from build123d import *

# Parameters (mm, degrees)
SKETCH1_R           = 23.87
SKETCH1_R_2         = 1.5875
SKETCH1_R_3         = 1.3208
SKETCH1_R_4         = 4
BOSS_EXTRUDE2_DEPTH = 1.016


with BuildPart() as part:
    # Sketch1 → Boss-Extrude2 (new body)
    with BuildSketch(Plane.XY):
        Circle(SKETCH1_R)
        with Locations((0, 10)):
            Circle(SKETCH1_R_2, mode=Mode.SUBTRACT)
        with Locations((9.878281733, -9.878281733)):
            Circle(SKETCH1_R_3, mode=Mode.SUBTRACT)
        with Locations((9.878281733, 9.878281733)):
            Circle(SKETCH1_R_3, mode=Mode.SUBTRACT)
        with Locations((-9.878281733, -9.878281733)):
            Circle(SKETCH1_R_3, mode=Mode.SUBTRACT)
        with Locations((-9.878281733, 9.878281733)):
            Circle(SKETCH1_R_3, mode=Mode.SUBTRACT)
        Circle(SKETCH1_R_4, mode=Mode.SUBTRACT)
        with Locations((0, -10)):
            Circle(SKETCH1_R_2, mode=Mode.SUBTRACT)
    extrude(amount=BOSS_EXTRUDE2_DEPTH)


solid = part.part
The listing builds one solid part. Answer for the finished solid, in the listing's coordinates (mm). Round coordinates to 2 decimals unless told otherwise and drop trailing zeros. Write each loop counter-clockwise with the first axis right and the second up, starting at its lowest first coordinate (ties: lowest second). Pieces come first, ordered by that corner, then holes. Notation, with made-up numbers: (15.5, 38.25) - (29.5, 38.25) arc R17 cw to (29.5, 59.25) - close; hole circle Ø8 at (65.25, 82). An arc over 180 degrees is marked (long way). Use one line per item in the form item = value. Start each with the question number.
Item 1: A cutting plane is placed at C-C (z = 0.8). Write down the section's boundary in (x, y) (1 decimal).
Item 2: A cutting plane is placed at A-A (x = 0). Write down the section's boundary in (y, z).
Item 3: A cutting plane is placed at D-D (y = -13). Write down the section's boundary in (x, z), plus the area to 3 significant figures.
Item 4: Determine the mould class of faces 1 (the cylindrical face through (0.73, 8.59, 0.5)), 2 (the cylindrical face through (-3.107, 23.667, 0.501)), 3 (the flat face through (5, 0, 1.016)) for opening direction X: +X half, -X half, draft (parallel to the pull), parting line (faces both ways), or undercut.
Item 5: Find the intervals of material crossed by line 1 (Y direction, x = 0, z = 0.2); line 2 (Y direction, x = -1, z = 0.5); line 3 (X direction, y = 9, z = 0.65), in increasing order. Write a range as [from, to].
Item 6: A cutting plane is placed at B-B (y = 0). Write down the section's boundary in (x, z), plus the area to 3 significant figures.
The answers:
q1.outline = circle Ø47.7 at (0, 0); hole circle Ø2.6 at (-9.9, -9.9); hole circle Ø2.6 at (-9.9, 9.9); hole circle Ø8 at (0, 0); hole circle Ø3.2 at (0, -10); hole circle Ø3.2 at (0, 10); hole circle Ø2.6 at (9.9, -9.9); hole circle Ø2.6 at (9.9, 9.9)
q2.outline = (-23.87, 0) - (-11.59, 0) - (-11.59, 1.02) - (-23.87, 1.02) - close; (-8.41, 0) - (-4, 0) - (-4, 1.02) - (-8.41, 1.02) - close; (4, 0) - (8.41, 0) - (8.41, 1.02) - (4, 1.02) - close; (11.59, 0) - (23.87, 0) - (23.87, 1.02) - (11.59, 1.02) - close
q3.outline = (-20.02, 0) - (20.02, 0) - (20.02, 1.02) - (-20.02, 1.02) - close
q3.area = 40.7 mm^2
q4.face_1 = undercut
q4.face_2 = parting line
q4.face_3 = draft
q5.line_1 = [-23.87, -11.59], [-8.41, -4], [4, 8.41], [11.59, 23.87]
q5.line_2 = [-23.85, -11.23], [-8.77, -3.87], [3.87, 8.77], [11.23, 23.85]
q5.line_3 = [-22.11, -10.86], [-8.89, -1.23], [1.23, 8.89], [10.86, 22.11]
q6.outline = (-23.87, 0) - (-4, 0) - (-4, 1.02) - (-23.87, 1.02) - close; (4, 0) - (23.87, 0) - (23.87, 1.02) - (4, 1.02) - close
q6.area = 40.4 mm^2
